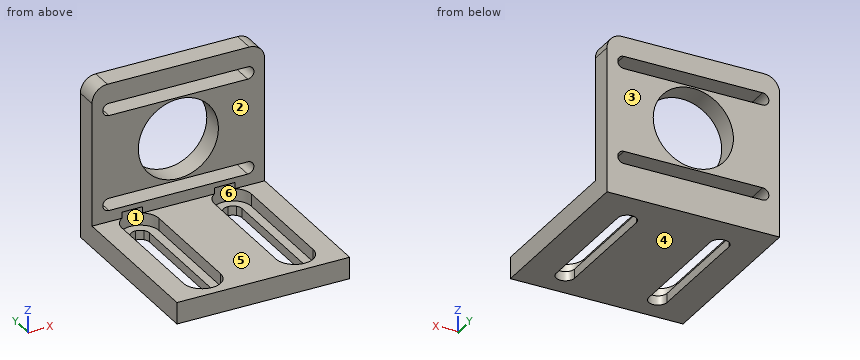
```python
from build123d import *

# Parameters (mm, degrees)
ESBO_O1_W                  = 56
ESBO_O1_H                  = 58
RESSALTO_EXTRUS_O1_DEPTH   = 7
CORTE_EXTRUS_O1_DEPTH      = 7
ESBO_O4_W                  = 56
ESBO_O4_H                  = 7
RESSALTO_EXTRUS_O2_DEPTH   = 45
ESBO_O5_R                  = 13
ESBO_O5_R_2                = 2
CORTE_EXTRUS_O2_DEPTH      = 45
CORTE_EXTRUS_O3_DEPTH      = 2
CORTE_EXTRUS_O3_DEPTH_BACK = 4
FILETE1_R                  = 5
CORTE_EXTRUS_O4_DEPTH      = 10


with BuildPart() as part:
    # Esboço1 → Ressalto-extrusão1 (new body)
    with BuildSketch(Plane.XY):
        with Locations((-35.670310893, 154.468429513)):
            Rectangle(ESBO_O1_W, ESBO_O1_H)
    extrude(amount=RESSALTO_EXTRUS_O1_DEPTH)

    # Esboço3 → Corte-extrusão1 (cut)
    with BuildSketch(Plane.XY.offset(7)):
        with BuildLine():
            Line((-47.670310893, 134.468429513), (-47.670310893, 171.468429513))
            ThreePointArc((-47.670310893, 171.468429513), (-47.867793816, 172.538895782), (-48.434242916, 173.468429513))
            ThreePointArc((-48.434242916, 173.468429513), (-49.445566022, 174.2070423), (-50.670310893, 174.468429513))
            ThreePointArc((-50.670310893, 174.468429513), (-51.895055765, 174.2070423), (-52.906378871, 173.468429513))
            ThreePointArc((-52.906378871, 173.468429513), (-53.47282797, 172.538895782), (-53.670310893, 171.468429513))
            Line((-53.670310893, 171.468429513), (-53.670310893, 134.468429513))
            ThreePointArc((-53.670310893, 134.468429513), (-50.670310893, 131.468429513), (-47.670310893, 134.468429513))
        make_face()
        with BuildLine():
            Line((-23.670310893, 171.468429513), (-23.670310893, 134.468429513))
            ThreePointArc((-23.670310893, 134.468429513), (-20.670310893, 131.468429513), (-17.670310893, 134.468429513))
            Line((-17.670310893, 134.468429513), (-17.670310893, 171.468429513))
            ThreePointArc((-17.670310893, 171.468429513), (-17.867793816, 172.538895782), (-18.434242916, 173.468429513))
            ThreePointArc((-18.434242916, 173.468429513), (-19.445566022, 174.2070423), (-20.670310893, 174.468429513))
            ThreePointArc((-20.670310893, 174.468429513), (-21.895055765, 174.2070423), (-22.906378871, 173.468429513))
            ThreePointArc((-22.906378871, 173.468429513), (-23.47282797, 172.538895782), (-23.670310893, 171.468429513))
        make_face()
    extrude(amount=-CORTE_EXTRUS_O1_DEPTH, mode=Mode.SUBTRACT)

    # Esboço4 → Ressalto-extrusão2 (add)
    with BuildSketch(Plane.XY.offset(7)):
        with Locations((-35.670310893, 179.968429513)):
            Rectangle(ESBO_O4_W, ESBO_O4_H)
    extrude(amount=RESSALTO_EXTRUS_O2_DEPTH)

    # Esboço5 → Corte-extrusão2 (cut)
    with BuildSketch(Plane.XZ.offset(-176.468429513)):
        with Locations((-35.670310893, 28.15)):
            Circle(ESBO_O5_R)
        with Locations((-51.170310893, 43.65)):
            Circle(ESBO_O5_R_2)
        with Locations((-20.170310893, 43.65)):
            Circle(ESBO_O5_R_2)
        with Locations((-51.170310893, 12.65)):
            Circle(ESBO_O5_R_2)
        with Locations((-20.170310893, 12.65)):
            Circle(ESBO_O5_R_2)
    extrude(amount=-CORTE_EXTRUS_O2_DEPTH, mode=Mode.SUBTRACT)

    # Esboço6 → Corte-extrusão3 (cut, two sides)
    with BuildSketch(Plane.XY.offset(7)) as corte_extrus_o3_sk:
        with BuildLine():
            Line((-56.670310893, 171.468429513), (-56.670310893, 134.468429513))
            ThreePointArc((-56.670310893, 134.468429513), (-50.670310893, 128.468429513), (-44.670310893, 134.468429513))
            Line((-44.670310893, 134.468429513), (-44.670310893, 171.468429513))
            ThreePointArc((-44.670310893, 171.468429513), (-50.670310893, 177.468429513), (-56.670310893, 171.468429513))
        make_face()
        with BuildLine():
            Line((-14.670310893, 134.468429513), (-14.670310893, 171.468429513))
            ThreePointArc((-14.670310893, 171.468429513), (-20.670310893, 177.468429513), (-26.670310893, 171.468429513))
            Line((-26.670310893, 171.468429513), (-26.670310893, 134.468429513))
            ThreePointArc((-26.670310893, 134.468429513), (-20.670310893, 128.468429513), (-14.670310893, 134.468429513))
        make_face()
    extrude(amount=CORTE_EXTRUS_O3_DEPTH, mode=Mode.SUBTRACT)
    extrude(corte_extrus_o3_sk.sketch, amount=-CORTE_EXTRUS_O3_DEPTH_BACK, mode=Mode.SUBTRACT)

    # Filete1
    filete1_edges = [part.edges().sort_by_distance(p)[0] for p in [
        (-63.670310893, 179.968429513, 52),
        (-7.670310893, 179.968429513, 52),
    ]]
    fillet(filete1_edges, radius=FILETE1_R)

    # Esboço7 → Corte-extrusão4 (cut)
    with BuildSketch(Plane(origin=(0, 183.468429513, 0), x_dir=(1, 0, 0), z_dir=(0, 1, 0))):
        with BuildLine():
            Line((-58.170310893, -10.65), (-13.170310893, -10.65))
            ThreePointArc((-13.170310893, -10.65), (-11.170310893, -12.65), (-13.170310893, -14.65))
            Line((-13.170310893, -14.65), (-58.170310893, -14.65))
            ThreePointArc((-58.170310893, -14.65), (-60.170310893, -12.65), (-58.170310893, -10.65))
        make_face()
        with BuildLine():
            Line((-13.170310893, -45.65), (-58.170310893, -45.65))
            ThreePointArc((-58.170310893, -45.65), (-60.170310893, -43.65), (-58.170310893, -41.65))
            Line((-58.170310893, -41.65), (-13.170310893, -41.65))
            ThreePointArc((-13.170310893, -41.65), (-11.170310893, -43.65), (-13.170310893, -45.65))
        make_face()
    extrude(amount=-CORTE_EXTRUS_O4_DEPTH, mode=Mode.SUBTRACT)


solid = part.part
```
Geometry check sheet. Reference: the model listing, model coordinates, mm. Face numbers are marked on the shaded views. A direction names the side the tool comes from. Give positions to 0.01 mm unless a question says otherwise; leave off trailing zeros. Order: outer loops, then holes, each group sorted by start corner. A loop starts at its lowest first (then second) coordinate and runs counter-clockwise, first axis right, second up.
1. Gauge pin test, flat ends, axial feed: pin 1 Ø1 at (x, z) = (-17, 34.5) entering from -Y; pin 2 Ø10 at (x, y) = (-25, 142.5) entering from +Z. Record the tip position at first contact, or that the pin passes through.
2. Section check B-B, the plane y = 138. Enter the section's corners in (x, z), and give its area (3 significant figures).
3. Thickness scan on L1, parallel to Z at x = -50.5, y = 178; L2, parallel to X at y = 145, z = 4; L3, parallel to X at y = 180, z = 28. Record the ranges inside material, lowest first.
4. Access from +Z, -Z, +X, -X, +Y, -Y to the whole of each face (thin tool, end or side, straight path). Record for the marked faces 1, 2 and 3.
5. Section check A-A, the plane z = 28.15. Enter the section's corners in (x, y).
6. Release check for a two-part mould opening along Z. For the marked faces 4, 5 and 6 record: pulls with the +Z half, pulls with the -Z half, needs draft (parallel to the pull), parting line crosses it, or undercut.
7. Section check C-C, the plane z = 12.65. Enter the section's corners in (x, y).
Values follow:
1. pin 1: stops at y = 176.47
1. pin 2: stops at z = 7
2. outline: (-63.67, 0) - (-53.67, 0) - (-53.67, 3) - (-56.67, 3) - (-56.67, 7) - (-63.67, 7) - close; (-47.67, 0) - (-23.67, 0) - (-23.67, 3) - (-26.67, 3) - (-26.67, 7) - (-44.67, 7) - (-44.67, 3) - (-47.67, 3) - close; (-17.67, 0) - (-7.67, 0) - (-7.67, 7) - (-14.67, 7) - (-14.67, 3) - (-17.67, 3) - close
2. area: 260 mm2
3. L1: z = 0 to 10.65, 14.65 to 41.65, 45.65 to 52
3. L2: x = -63.67 to -56.67, -44.67 to -26.67, -14.67 to -7.67
3. L3: x = -63.67 to -48.67, -22.67 to -7.67
4. face 1: none
4. face 2: +Z, +X, -X, -Y
4. face 3: +Z, -Z, +X, -X, +Y
5. outline: (-63.67, 176.47) - (-48.67, 176.47) - (-48.67, 183.47) - (-63.67, 183.47) - close; (-22.67, 176.47) - (-7.67, 176.47) - (-7.67, 183.47) - (-22.67, 183.47) - close
6. face 4: pulls with the -Z half
6. face 5: pulls with the +Z half
6. face 6: undercut
7. outline: (-63.67, 176.47) - (-60.17, 176.47) - (-60.17, 183.47) - (-63.67, 183.47) - close; (-11.17, 176.47) - (-7.67, 176.47) - (-7.67, 183.47) - (-11.17, 183.47) - close
